Could you check a few things on this model? Use its own coordinates, in mm. A direction names the side the tool comes from. Round coordinates to 2 decimals unless told otherwise and drop trailing zeros. Write each loop counter-clockwise with the first axis right and the second up, starting at its lowest first coordinate (ties: lowest second). Pieces come first, ordered by that corner, then holes. Notation, with made-up numbers: (50.5, 22.25) -> (97.5, 22.25) arc R32 ccw to (97.5, 53.25) -> close; hole circle Ø6 at (-20, -21.75). An arc over 180 degrees is marked (long way). Answer in a Markdown table with one row per item.
from build123d import *

# Parameters (mm, degrees)
F0_R      = 10
F1_DEPTH  = 21
F2_R      = 7.5
F3_DEPTH  = 4
F4_R      = 3
F5_DEPTH  = 1
F6_R      = 1
F7_R      = 1
F8_R      = 1
F9_R      = 1
F10_DEPTH = 9
F11_R     = 0.25
F12_W     = 0.5
F12_H     = 3
F13_DEPTH = 6
F14_R     = 1
F15_DEPTH = 3
F16_R     = 1
F17_DEPTH = 3
F18_R     = 0.75
F19_R     = 0.75


with BuildPart() as f1:
    # F0 (on Top) → F1 (new body)
    with BuildSketch(Plane.XY):
        Circle(F0_R)
    extrude(amount=F1_DEPTH)

    # F2 (on face) → F3 (join)
    with BuildSketch(Plane.XY.offset(21)):
        Circle(F2_R)
    extrude(amount=F3_DEPTH)

    # F4 (on face) → F5 (join)
    with BuildSketch(Plane.XY.offset(25)):
        Circle(F4_R)
    extrude(amount=F5_DEPTH)

    # F6
    f6_edges = [f1.edges().sort_by_distance(p)[0] for p in [
        (-10, 0, 0),
    ]]
    fillet(f6_edges, radius=F6_R)

    # F7
    f7_edges = [f1.edges().sort_by_distance(p)[0] for p in [
        (-10, 0, 21),
    ]]
    fillet(f7_edges, radius=F7_R)

    # F8
    f8_edges = [f1.edges().sort_by_distance(p)[0] for p in [
        (-7.5, 0, 25),
    ]]
    fillet(f8_edges, radius=F8_R)

    # F9 (on face) → F10 (join)
    with BuildSketch(Plane.XY.offset(26)):
        Circle(F9_R)
    extrude(amount=F10_DEPTH)

    # F11
    f11_edges = [f1.edges().sort_by_distance(p)[0] for p in [
        (-1, 0, 35),
    ]]
    fillet(f11_edges, radius=F11_R)

    # F12 (on face) → F13 (join)
    with BuildSketch(Plane(origin=(0, 0, 0), x_dir=(1, 0, 0), z_dir=(0, 0, -1))):
        with Locations((-7.267895, -0.302635)):
            Rectangle(F12_W, F12_H)
        with Locations((5.892853, -0.302635)):
            Rectangle(F12_W, F12_H)
    extrude(amount=F13_DEPTH)

    # F14 (on face) → F15 (cut)
    with BuildSketch(Plane(origin=(-7.517895, 0, 0), x_dir=(0, -1, 0), z_dir=(-1, 0, 0))):
        with Locations((-0.34836, -4)):
            Circle(F14_R)
    extrude(amount=-F15_DEPTH, mode=Mode.SUBTRACT)

    # F16 (on face) → F17 (cut)
    with BuildSketch(Plane.YZ.offset(6.142853)):
        with Locations((0.362238, -4)):
            Circle(F16_R)
    extrude(amount=-F17_DEPTH, mode=Mode.SUBTRACT)

    # F18
    f18_edges = [f1.edges().sort_by_distance(p)[0] for p in [
        (-7.267895, -1.197365, -6),
        (-7.267895, 1.802635, -6),
    ]]
    fillet(f18_edges, radius=F18_R)

    # F19
    f19_edges = [f1.edges().sort_by_distance(p)[0] for p in [
        (5.892853, -1.197365, -6),
        (5.892853, 1.802635, -6),
    ]]
    fillet(f19_edges, radius=F19_R)


solid = f1.part
1) Imagine slicing it at D-D, the plane y = 0. Count the separate pieces of the cut face and the enclosed holes in it, plus the area to 3 significant figures.
Findings:
| item | result |
|---|---|
| separate pieces | 3 |
| enclosed holes | 0 |
| area | 507 mm^2 |
2) Imagine slicing it at A-A, the plane z = -4. Please give me the cut outline in (x, y), plus the area to 4 significant figures.
Findings:
| item | result |
|---|---|
| outline | (-7.52, -1.2) -> (-7.02, -1.2) -> (-7.02, -0.65) -> (-7.52, -0.65) -> close; (-7.52, 1.35) -> (-7.02, 1.35) -> (-7.02, 1.8) -> (-7.52, 1.8) -> close; (5.64, -1.2) -> (6.14, -1.2) -> (6.14, -0.64) -> (5.64, -0.64) -> close; (5.64, 1.36) -> (6.14, 1.36) -> (6.14, 1.8) -> (5.64, 1.8) -> close |
| area | 1.000 mm^2 |
3) Please list where these lines run through material, in increasing order: line 1 (Z direction, x = 4.5, y = -1); line 2 (X direction, y = 0.5, z = 29.5); line 3 (X direction, y = -6.5, z = 18).
Findings:
| item | result |
|---|---|
| line 1 | z = 0 to 25 |
| line 2 | x = -0.87 to 0.87 |
| line 3 | x = -7.6 to 7.6 |
4) For pin 1 (8 mm diameter, centred on y = 5, z = 3.5, fed in from +X); pin 2 (5 mm diameter, centred on x = 6.5, z = 25.5, fed in from +Y); pin 3 (10 mm diameter, centred on x = -8, y = 1.5, fed in from +Z), each with a flat end and sliding along its axis, tell me the tip position at first contact or that it passes through.
Findings:
| item | result |
|---|---|
| pin 1 | stops at x = 9.95 |
| pin 2 | stops at y = 6.08 |
| pin 3 | stops at z = 25 |
5) For faces 4 (the face through (-7.518, 1, -3)), 5 (the face through (6.143, 1, -3)), 6 (the face through (3, -1, 25)), 7 (the face through (-7.018, 1, -3)), which set-ups out of +Z, -Z, +X, -X, +Y, -Y let a thin tool reach every point of the face, with its end or its side?
Findings:
| item | result |
|---|---|
| face 4 | -Z, -X, +Y, -Y |
| face 5 | -Z, +X, +Y, -Y |
| face 6 | +Z |
| face 7 | -Z, +Y, -Y |
6) Imagine slicing it at B-B, the plane x = 0. Please give me the cut outline in (y, z), plus the area to 3 significant figures.
Findings:
| item | result |
|---|---|
| outline | (-10, 1) arc R1 ccw to (-9, 0) -> (9, 0) arc R1 ccw to (10, 1) -> (10, 20) arc R1 ccw to (9, 21) -> (7.5, 21) -> (7.5, 24) arc R1 ccw to (6.5, 25) -> (3, 25) -> (3, 26) -> (1, 26) -> (1, 34.75) arc R0.25 ccw to (0.75, 35) -> (-0.75, 35) arc R0.25 ccw to (-1, 34.75) -> (-1, 26) -> (-3, 26) -> (-3, 25) -> (-6.5, 25) arc R1 ccw to (-7.5, 24) -> (-7.5, 21) -> (-9, 21) arc R1 ccw to (-10, 20) -> close |
| area | 503 mm^2 |
7) Thinking about a two-plate mould opening in Z: for faces 1 (the face through (-3, 0.1, 25.5)), 2 (the face through (-7.27, 0.48, -3.01)), 3 (the face through (-2, 7.4, 21)), which applies, +Z half, -Z half, draft (parallel to the pull), parting line (faces both ways), or undercut?
Findings:
| item | result |
|---|---|
| face 1 | draft |
| face 2 | undercut |
| face 3 | +Z half |
8) Imagine slicing it at C-C, the plane z = 8.5. Please give me the cut outline in (x, y).
Findings:
| item | result |
|---|---|
| outline | circle Ø20 at (0, 0) |
